Design review of the part built by this model. Coordinates are the model's own, in mm. Face numbers are marked on the shaded views. A direction names the side the tool comes from. Coordinates: 2 decimals unless noted, no trailing zeros. Loops run counter-clockwise (first coordinate to the right, second up) from the corner with the lowest first, then second, coordinate; pieces in that order, holes last. Notation, with made-up numbers: (-26, 69) -> (14, 69) arc R14 ccw to (14, 90) -> close; hole circle Ø1 at (86, 31). An arc over 180 degrees is marked (long way). Answer in a Markdown table with one row per item.
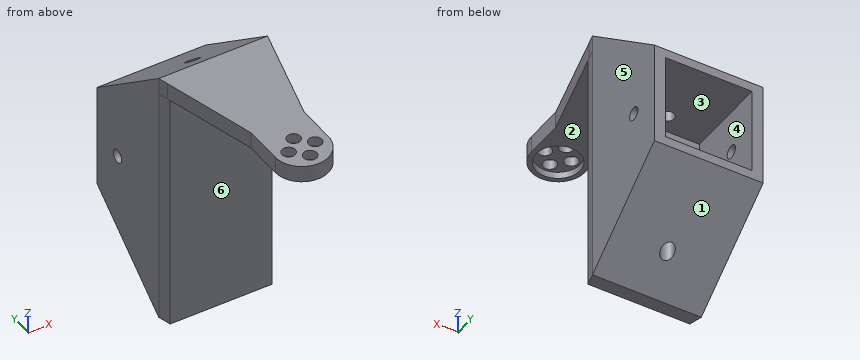
Autodesk Inventor part; units mm, degrees
ref_plane "Work Plane1" through (0, 0, 2.5) normal (0, 0, 1) x (1, 0, 0)
ref_plane "YZ Plane" through (0, 0, 0) normal (1, 0, 0) x (0, 1, 0)
ref_plane "XZ Plane" through (0, 0, 0) normal (0, 1, 0) x (-1, 0, 0)
sketch "Sketch1" plane through (0, 0, 0) normal (0, 0, 1) x (1, 0, 0)
  circle A0 centre (0, 4) radius 2
  circle A1 centre (-4, 0) radius 2
  circle A2 centre (0, -4) radius 2
  circle A3 centre (4, 0) radius 2
  line L0 (8, 11.7321) -> (15.5744, 40)
  line L1 (7, 8) -> (40.1288, 8) construction
  line L2 (-8, 11.7321) -> (-15.5744, 40)
  line L3 (8, 0) -> (8, 11.7321)
  line L4 (-8, 0) -> (-8, 11.7321)
  arc A4 (-8, 0) -> (8, 0) centre (0, 0) ccw
  line L5 (0, 43) -> (16.3782, 43)
  line L6 (16.3782, 43) -> (15.5744, 40)
  line L7 (-15.5744, 40) -> (-16.3782, 43)
  line L8 (-16.3782, 43) -> (0, 43)
  dimension "d2" = 4
  dimension "d5" = 360
extrude "Extrusion1" add sketch "Sketch1" along normal blind 5
sketch "Sketch2" plane through (0, 0, 0) normal (0, 0, -1) x (-1, 0, 0)
  circle A0 centre (0, 0) radius 6.625
  dimension "d18" = 13.25
extrude "Extrusion2" cut sketch "Sketch2" against normal blind 2
sketch "Sketch4" plane through (0, 0, 0) normal (0, 0, -1) x (-1, 0, 0)
  line L0 (-8, 11.7321) -> (-16.3782, 43)
  line L1 (-16.3782, 43) -> (16.3782, 43)
  line L2 (-16.3782, 43) -> (16.3782, 43)
  line L3 (0, 39.136) -> (15.3429, 39.136)
  line L4 (16.3782, 43) -> (8, 11.7321)
  line L5 (15.3429, 39.136) -> (16.3782, 43)
  line L6 (0, 39.136) -> (-15.3429, 39.136)
  line L7 (-15.3429, 39.136) -> (-16.3782, 43)
  point P0 (0, 0)
extrude "Extrusion4" add sketch "Sketch4" along normal blind 73.5
sketch "Sketch5" plane through (-16.3782, 43, 5) normal (0, 1, 0) x (1, 0, 0)
  line L0 (0, 78.5) -> (32.7564, 78.5)
  line L1 (32.7564, 0) -> (0, 0)
  line L2 (0, 78.5) -> (32.7564, 78.5)
  line L3 (32.7564, 78.5) -> (32.7564, 0)
  line L4 (32.7564, 0) -> (0, 0)
  line L5 (0, 0) -> (0, 78.5)
  point P0 (16.3782, 5)
extrude "Extrusion5" add sketch "Sketch5" along normal blind 30
sketch "Sketch6" plane through (16.3782, 43, -73.5) normal (1, 0, 0) x (0, 0, -1)
  line L0 (-78.5, 30) -> (0, 30)
  line L1 (-39.25, 30) -> (-26.55, 30)
  line L2 (-39.25, 30) -> (-51.95, 30)
  line L3 (-51.95, 30) -> (-54.95, 30)
  line L4 (-26.55, 30) -> (-23.55, 30)
  line L5 (0, -3.864) -> (0, 0)
  line L6 (-23.55, 30) -> (0, 0)
  line L7 (0, 0) -> (0, 30)
  line L8 (0, 0) -> (0, 30)
  line L9 (0, 30) -> (-23.55, 30)
  line L10 (-54.95, 30) -> (-78.5, 30)
  line L11 (-78.5, 0) -> (-78.5, 30)
  line L12 (-78.5, 30) -> (-78.5, 0)
  line L13 (-78.5, 0) -> (-54.95, 30)
  point P0 (-73.5, -43)
  dimension "d30" = 12.7
  dimension "d31" = 12.7
  dimension "d32" = 3
  dimension "d33" = 3
extrude "Extrusion6" cut sketch "Sketch6" against normal up to surface (32.7564 mm away)
sketch "Sketch7" plane through (-16.3782, 73, 5) normal (0, 1, 0) x (1, 0, 0)
  line L0 (0, 78.5) -> (0, 0)
  line L1 (0, 23.55) -> (32.7564, 23.55)
  line L2 (16.3782, 52.25) -> (3.3782, 52.25)
  line L3 (3.3782, 52.25) -> (3.3782, 26.25)
  line L4 (3.3782, 26.25) -> (29.3782, 26.25)
  line L5 (29.3782, 26.25) -> (29.3782, 52.25)
  line L6 (29.3782, 52.25) -> (16.3782, 52.25)
  point P0 (16.3782, 5)
  dimension "d37" = 13
  dimension "d38" = 26
  dimension "d39" = 26
extrude "Extrusion7" cut sketch "Sketch7" against normal blind 25.4
ref_plane "Work Plane1" through (0, 0, 2.5) normal (0, 0, 1) x (1, 0, 0)
sketch "Sketch8" plane through (0, 0, 2.5) normal (0, 0, 1) x (1, 0, 0)
  line L0 (16.3782, 43) -> (-16.3782, 43)
  circle A0 centre (0, 53) radius 2
  point P0 (0, 0)
  dimension "d43" = 4
extrude "Extrusion8" cut sketch "Sketch8" against normal through all
sketch "Sketch9" plane through (16.3782, 43, 5) normal (1, 0, 0) x (0, 0, -1)
  line L0 (26.25, 30) -> (52.25, 30)
  circle A0 centre (39.25, 20) radius 2
  point P0 (5, -43)
  dimension "d47" = 4
extrude "Extrusion9" cut sketch "Sketch9" against normal up to surface (32.7564 mm away)
properties part number "OutPut_Shaft_From_Gearbox"
(1) For pin 1 (13 mm diameter, centred on x = 3, z = -29, fed in from +Y); pin 2 (7.5 mm diameter, centred on x = 1.5, y = 55.5, fed in from +Z); pin 3 (5 mm diameter, centred on x = 0, y = 53, fed in from -Z), all flat-tipped, find the tip position at first contact; note any pin that passes through.
Evaluation:
| item | result |
|---|---|
| pin 1 | stops at y = 47.6 |
| pin 2 | stops at z = -1.87 |
| pin 3 | stops at z = -67.61 |
(2) Take a section at A-A on y = 63. Give the boundary of the cut face in (x, z), and give its area (3 significant figures).
Evaluation:
| item | result |
|---|---|
| outline | (-16.38, -57.8) -> (16.38, -57.8) -> (16.38, -36.25) -> (13, -36.25) -> (13, -47.25) -> (-13, -47.25) -> (-13, -36.25) -> (-16.38, -36.25) -> close; (-16.38, -32.25) -> (-13, -32.25) -> (-13, -21.25) -> (13, -21.25) -> (13, -32.25) -> (16.38, -32.25) -> (16.38, -10.7) -> (-16.38, -10.7) -> close |
| area | 840 mm² |
(3) Take a section at C-C on z = -20. Give the boundary of the cut face in (x, y), and give its area (3 significant figures).
Evaluation:
| item | result |
|---|---|
| outline | (-16.38, 43) -> (-15.34, 39.14) -> (15.34, 39.14) -> (16.38, 43) -> (16.38, 73) -> (-16.38, 73) -> close; hole circle Ø4 at (0, 53) |
| area | 1,090 mm² |
(4) Draft analysis for pull direction X (two halves, no side actions). For the marked faces 4, 5 and 6, state which applies: pulls with the +X half, pulls with the -X half, needs draft (parallel to the pull), parting line crosses it, or undercut.
Evaluation:
| item | result |
|---|---|
| face 4 | undercut |
| face 5 | pulls with the +X half |
| face 6 | needs draft |
(5) Take a section at B-B on y = 1. Give the boundary of the cut face in (x, z), and give its area (3 significant figures).
Evaluation:
| item | result |
|---|---|
| outline | (-8, 0) -> (-6.55, 0) -> (-6.55, 2) -> (-5.73, 2) -> (-5.73, 5) -> (-8, 5) -> close; (-2.27, 2) -> (2.27, 2) -> (2.27, 5) -> (-2.27, 5) -> close; (5.73, 2) -> (6.55, 2) -> (6.55, 0) -> (8, 0) -> (8, 5) -> (5.73, 5) -> close |
| area | 33.0 mm² |
(6) Take a section at D-D on x = -4. Give the boundary of the cut face in (y, z), and give its area (3 significant figures).
Evaluation:
| item | result |
|---|---|
| outline | (-6.93, 0) -> (-5.28, 0) -> (-5.28, 2) -> (-2, 2) -> (-2, 5) -> (-6.93, 5) -> close; (2, 2) -> (5.28, 2) -> (5.28, 0) -> (39.14, 0) -> (39.14, -73.5) -> (43, -73.5) -> (73, -49.95) -> (73, -47.25) -> (47.6, -47.25) -> (47.6, -21.25) -> (73, -21.25) -> (73, -18.55) -> (43, 5) -> (2, 5) -> close |
| area | 1,490 mm² |
(7) To check wall thickness, follow probe 1 along X at (y, z) = (0, 4); probe 2 along Y at (x, z) = (15, -34); probe 3 along X at (y, z) = (59, -33.5). State the ranges of each line that lie inside material, in increasing order.
Evaluation:
| item | result |
|---|---|
| probe 1 | x = -8 to -6, -2 to 2, 6 to 8 |
| probe 2 | y = 39.14 to 61.02, 64.98 to 73 |
| probe 3 | x = -16.38 to -13, 13 to 16.38 |
(8) Tool access review of the marked faces 1, 2 and 3: name each direction out of +Z, -Z, +X, -X, +Y, -Y from which nothing blocks a thin tool from reaching the whole face with its end or side.
Evaluation:
| item | result |
|---|---|
| face 1 | -Z, +X, -X, +Y |
| face 2 | -Z, +X, -X, -Y |
| face 3 | +Y |
